Geometry check sheet. Reference: the model listing, model coordinates, mm. Round coordinates to 2 decimals unless told otherwise and drop trailing zeros. Write each loop counter-clockwise with the first axis right and the second up, starting at its lowest first coordinate (ties: lowest second). Pieces come first, ordered by that corner, then holes. Notation, with made-up numbers: M 43,78 L 59,78 A34 ccw 59,113 Z; hole C -6,47 d2. An arc over 180 degrees is marked long. Put each result on its own line as item: value. Start each with the question number.
(1) Material ranges on probe 1 along Y at (x, z) = (-71.9, 4); probe 2 along X at (y, z) = (38, 3.5); probe 3 along X at (y, z) = (37, 5.75), recorded low to high.
(2) Section check A-A on x = -24.6. Record the cut outline in (y, z), then the cut area to 3 significant figures.
(3) Section check C-C on z = 1.25. Record the cut outline in (x, y), then the cut area to 3 significant figures.
(4) Section check B-B on y = 38.1. Record the cut outline in (x, z).
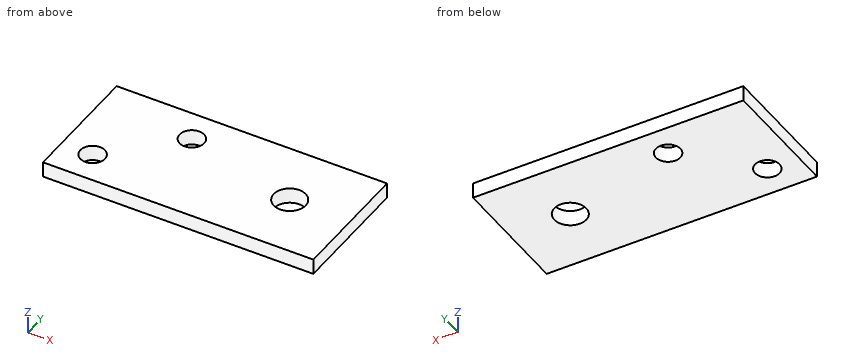
from build123d import *

# Parameters (mm, degrees)
CROQUIS1_R              = 6.501341754
SALIENTE_EXTRUIR1_DEPTH = 6.31
CROQUIS2_R              = 5
CORTAR_EXTRUIR1_DEPTH   = 10


with BuildPart() as part:
    # Croquis1 → Saliente-Extruir1 (new body)
    with BuildSketch(Plane.XY):
        Polygon((-59.2, 50.8), (-110, 50.8), (-110, 0), (0, 0), (0, 50.8), align=None)
        with Locations((-24.6, 25.401341754)):
            Circle(CROQUIS1_R, mode=Mode.SUBTRACT)
    extrude(amount=SALIENTE_EXTRUIR1_DEPTH)

    # Croquis2 → Cortar-Extruir1 (cut)
    with BuildSketch(Plane(origin=(0, 0, 0), x_dir=(-1, 0, 0), z_dir=(0, 0, -1))):
        with Locations((97.3, 12.7)):
            Circle(CROQUIS2_R)
        with Locations((71.9, 38.1)):
            Circle(CROQUIS2_R)
    extrude(amount=-CORTAR_EXTRUIR1_DEPTH, mode=Mode.SUBTRACT)


solid = part.part
Answers follow:
1. probe 1: y = 0 to 33.1, 43.1 to 50.8
1. probe 2: x = -110 to -76.9, -66.9 to 0
1. probe 3: x = -110 to -76.78, -67.02 to 0
2. outline: M 0,0 L 18.9,0 L 18.9,6.31 L 0,6.31 Z; M 31.9,0 L 50.8,0 L 50.8,6.31 L 31.9,6.31 Z
2. area: 239 mm^2
3. outline: M -110,0 L 0,0 L 0,50.8 L -110,50.8 Z; hole C -97.3,12.7 d10; hole C -71.9,38.1 d10; hole C -24.6,25.4 d13
3. area: 5,300 mm^2
4. outline: M -110,0 L -76.9,0 L -76.9,6.31 L -110,6.31 Z; M -66.9,0 L 0,0 L 0,6.31 L -66.9,6.31 Z
